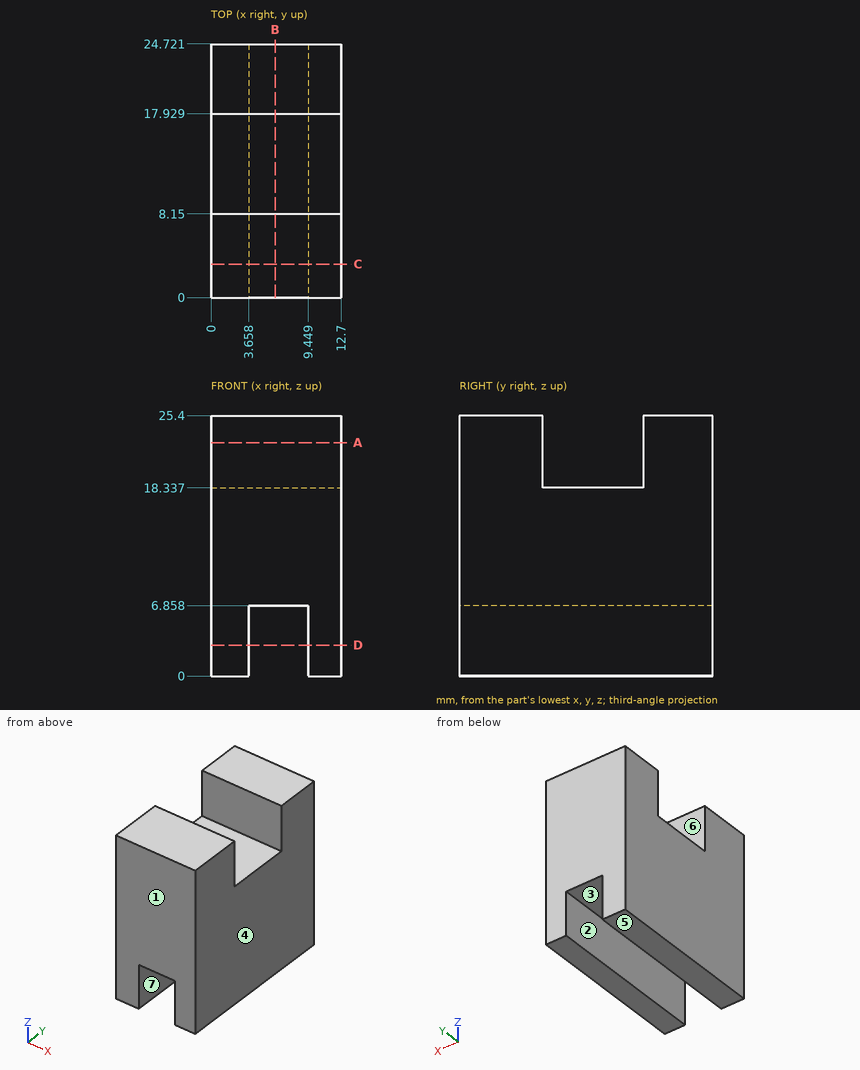
Check sheet for the drawn part. Datum: minimum x, y, z corner. Units: mm. A direction names the side the tool comes from. Round coordinates to 2 decimals unless told otherwise and drop trailing zeros. Loops run counter-clockwise (first coordinate to the right, second up) from the corner with the lowest first, then second, coordinate; pieces in that order, holes last. Notation, with made-up numbers: (71, -28) - (122, -28) arc R21 cw to (122, -21) - close; hole circle Ø6 at (22, 38.25). An arc over 180 degrees is marked (long way). Write item = value, one per line. Start each with the question number.
1. Section check D-D on z = 3. Enter the section's corners in (x, y), then the cut area to 3 significant figures.
2. Section check A-A on z = 22.75. Enter the section's corners in (x, y).
3. Set-up check for the marked faces 5, 6 and 7: record each of +Z, -Z, +X, -X, +Y, -Y from which the full face is reachable in a straight line by a thin tool's end or side.
4. Thickness scan on line 1 (Y direction, x = 3, z = 20); line 2 (X direction, y = 4.5, z = 4); line 3 (Z direction, x = 5, y = 4.25). Record the ranges inside material, lowest first.
5. Section check C-C on y = 3.25. Enter the section's corners in (x, z), then the cut area to 3 significant figures.
6. Mould release check, pull along X, two halves, no side actions. Record for the marked faces 1, 2, 3 and 4: released by +X, released by -X, zero draft, split by the parting line, or undercut.
7. Section check B-B on x = 6.25. Enter the section's corners in (y, z).
8. Depth check by flat-ended pin: pin 1 (2 mm diameter, centred on x = 4, y = 14.5, fed in from +Z); pin 2 (1.7 mm diameter, centred on x = 7.5, y = 15, fed in from -Z). Enter the tip coordinate at first touch or a pass-through.
Working result:
q1.outline = (0, 0) - (3.66, 0) - (3.66, 24.72) - (0, 24.72) - close; (9.45, 0) - (12.7, 0) - (12.7, 24.72) - (9.45, 24.72) - close
q1.area = 171 mm^2
q2.outline = (0, 0) - (12.7, 0) - (12.7, 8.15) - (0, 8.15) - close; (0, 17.93) - (12.7, 17.93) - (12.7, 24.72) - (0, 24.72) - close
q3.face_5 = -Z, +X, -X, +Y, -Y
q3.face_6 = +Z, +X, -X
q3.face_7 = -Z, +Y, -Y
q4.line_1 = 0 to 8.15, 17.93 to 24.72
q4.line_2 = 0 to 3.66, 9.45 to 12.7
q4.line_3 = 6.86 to 25.4
q5.outline = (0, 0) - (3.66, 0) - (3.66, 6.86) - (9.45, 6.86) - (9.45, 0) - (12.7, 0) - (12.7, 25.4) - (0, 25.4) - close
q5.area = 283 mm^2
q6.face_1 = zero draft
q6.face_2 = undercut
q6.face_3 = undercut
q6.face_4 = released by +X
q7.outline = (0, 6.86) - (24.72, 6.86) - (24.72, 25.4) - (17.93, 25.4) - (17.93, 18.34) - (8.15, 18.34) - (8.15, 25.4) - (0, 25.4) - close
q8.pin_1 = 18.34
q8.pin_2 = 6.86
